Here's the drawing with two shaded views (mm, measured from the low corner). I have some questions. A direction names the side the tool comes from. Coordinates: 2 decimals unless noted, no trailing zeros. Write each loop counter-clockwise with the first axis right and the second up, starting at its lowest first coordinate (ties: lowest second). Pieces come first, ordered by that corner, then holes.
Item 1: I'm going to push flat-ended pins straight in: pin 1 Ø23 at (x, z) = (31.75, 42.51) entering from -Y; pin 2 Ø6.5 at (x, y) = (33.5, 9.5) entering from -Z; pin 3 Ø1.5 at (x, y) = (38, 1.5) entering from -Z; pin 4 Ø6.5 at (x, z) = (38, 12.5) entering from +Y (3 decimals). Where does each tip first touch, or does it pass through?
Item 2: If we section it at C-C (x = 31.75): Count the separate pieces of the cut face and the enclosed holes in it.
Item 3: We'd pull the mould along Y, two halves only. Please class the marked faces 3, 4 and 5: +Y half, -Y half, draft (parallel to the pull), parting line (faces both ways), or undercut.
Item 4: If we section it at A-A (y = 7): Please give me the cut outline in (x, z).
Item 5: If we section it at D-D (x = 8.5): Please give me the cut outline in (y, z) (1 decimal).
Item 6: If I drill on line 1 (Z direction, x = 15, y = 4); line 2 (Y direction, x = 35.5, z = 67) (1 decimal); line 3 (X direction, y = 1.25, z = 34.5), over which ranges is the centre line in solid material (lowest first)?
Item 7: If we section it at B-B (z = 43.5): Please give me the cut outline in (x, y) (1 decimal).
Item 8: For the marked faces 1 and 2, which set-ups out of +Z, -Z, +X, -X, +Y, -Y let a thin tool reach every point of the face, with its end or its side?
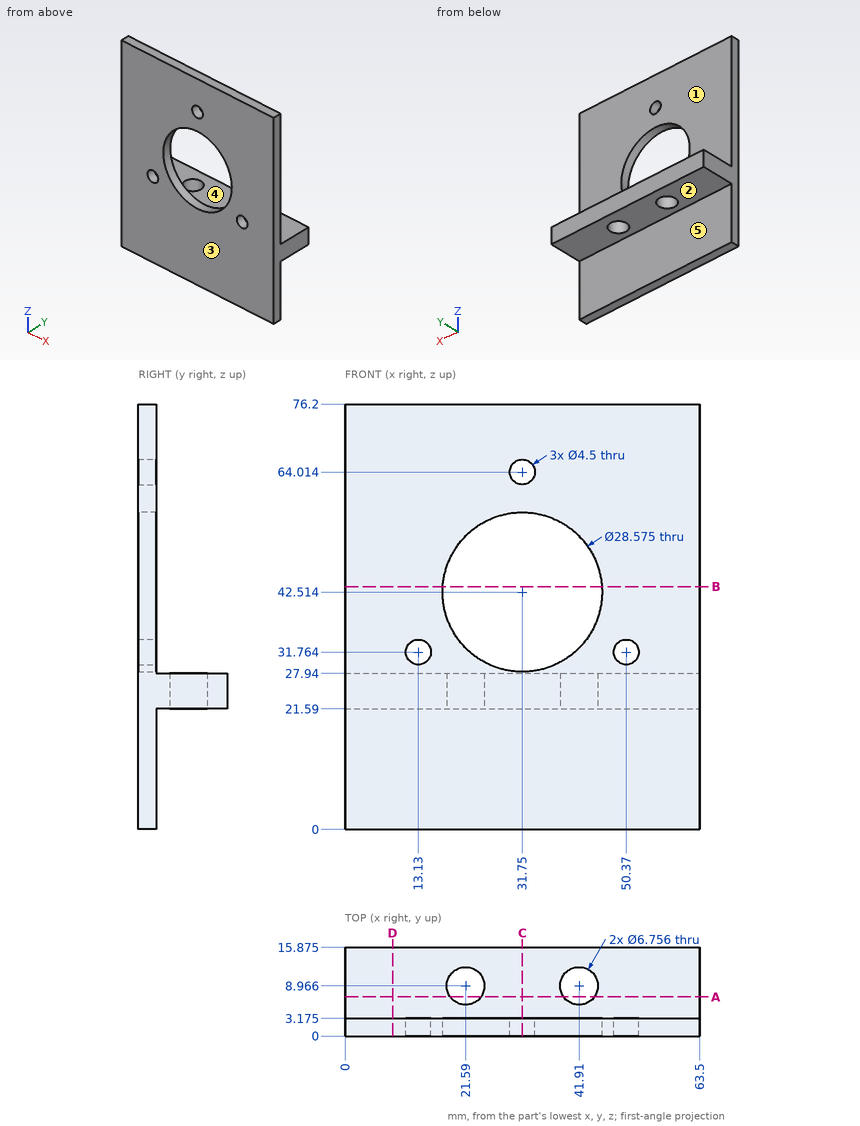
Answer list:
1. pin 1: passes through
1. pin 2: stops at z = 21.59
1. pin 3: stops at z = 0
1. pin 4: stops at y = 3.175
2. separate pieces: 3
2. enclosed holes: 0
3. face 3: -Y half
3. face 4: draft
3. face 5: +Y half
4. outline: (0, 21.59) - (18.84, 21.59) - (18.84, 27.94) - (0, 27.94) - close; (24.34, 21.59) - (39.16, 21.59) - (39.16, 27.94) - (24.34, 27.94) - close; (44.66, 21.59) - (63.5, 21.59) - (63.5, 27.94) - (44.66, 27.94) - close
5. outline: (0, 0) - (3.2, 0) - (3.2, 21.6) - (15.9, 21.6) - (15.9, 27.9) - (3.2, 27.9) - (3.2, 76.2) - (0, 76.2) - close
6. line 1: z = 21.59 to 27.94
6. line 2: y = 0 to 3.2
6. line 3: x = 0 to 19.92, 43.58 to 63.5
7. outline: (0, 0) - (17.5, 0) - (17.5, 3.2) - (0, 3.2) - close; (46, 0) - (63.5, 0) - (63.5, 3.2) - (46, 3.2) - close
8. face 1: +Z, +X, -X, +Y
8. face 2: -Z, +X, -X, +Y
